Here's how the part is built. I have some questions about the finished solid (model axes, mm). A direction names the side the tool comes from. Round coordinates to 2 decimals unless told otherwise and drop trailing zeros. Loops run counter-clockwise (first coordinate to the right, second up) from the corner with the lowest first, then second, coordinate; pieces in that order, holes last. Notation, with made-up numbers: (2.25, 19.5) -> (24.25, 19.5) arc R33 ccw to (24.25, 54.5) -> close; hole circle Ø3 at (88, -16.75). An arc over 180 degrees is marked (long way). Use one line per item in the form item = value. Start each with the question number.
Item 1: If we section it at A-A (y = 0): Write out the boundary of the cut face in (x, z) (3 decimals), then the cut area to 3 significant figures.
Item 2: If we section it at D-D (y = 18): Write out the boundary of the cut face in (x, z), then the cut area to 3 significant figures.
Item 3: I'm going to push flat-ended pins straight in: pin 1 Ø14 at (x, y) = (2, 1) entering from +Z; pin 2 Ø5 at (x, z) = (-7, 14) entering from -Y; pin 3 Ø12 at (x, y) = (-10.5, 3.5) entering from +Z; pin 4 Ø10 at (y, z) = (7.5, 9) entering from +X. Where does each tip first touch, or does it pass through?
Item 4: If we section it at B-B (z = 10.5): Write out the boundary of the cut face in (x, y).
Item 5: Thinking about a two-plate mould opening in Z: for faces 1 (the face through (0, -6, 0)), 2 (the face through (0, 25, 14)), 3 (the face through (18.567, 21.204, 19.586)), which applies, released by +Z, released by -Z, zero draft, split by the parting line, or undercut?
Item 6: If we section it at C-C (x = -20): Write out the boundary of the cut face in (y, z), then the cut area to 3 significant figures.
Item 7: For faces 4 (the face through (-24.57, -24.55, 2.79)), 5 (the face through (0, 17.3, 17)), which set-ups out of +Z, -Z, +X, -X, +Y, -Y let a thin tool reach every point of the face, with its end or its side?
Item 8: If I drill on L1, parallel to X at y = 20.5, z = 10.5; L2, parallel to X at y = 0, z = 4.3; L3, parallel to X at y = 9, z = 0.8 (3 decimals), over which ranges is the centre line in solid material (lowest first)? Write a range as [from, to].
Autodesk Fusion 360 part; units mm, degrees
sketch "Sketch1" plane through (0, 0, 0) normal (0, 0, 1) x (1, 0, 0)
  line L0 (25, 25) -> (-25, 25)
  line L1 (-25, 25) -> (-25, -25)
  line L2 (-25, -25) -> (25, -25)
  line L3 (25, -25) -> (25, 25)
  line L4 (25, 25) -> (-25, -25) construction
  line L5 (-25, 25) -> (25, -25) construction
  dimension "d1" = 50
  dimension "d2" = 50
extrude "Extrude1" add sketch "Sketch1" along normal blind 5.5
sketch "Sketch2" plane through (0, 0, 5.5) normal (0, 0, 1) x (-1, 0, 0)
  line L0 (-25, 25) -> (-25, -25)
  line L1 (-25, -25) -> (25, -25)
  line L2 (25, -25) -> (25, 25)
  line L3 (25, 25) -> (-25, 25)
  line L4 (25, -25) -> (-25, -25)
  line L5 (-25, -25) -> (-25, -17.3)
  line L6 (-25, -17.3) -> (25, -17.3)
  line L7 (25, -17.3) -> (25, -25)
  dimension "d11" = 7.7
  dimension "d12" = 50
extrude "Extrude2" add sketch "Sketch2" along normal blind 20 contours L0 L1 L2 L4 L5 L6 L7
sketch "Sketch3" plane through (0, 0, 5.5) normal (0, 0, 1) x (-1, 0, 0)
  line L0 (-25, -17.3) -> (25, -17.3)
  line L1 (25, -17.3) -> (25, 25)
  line L2 (25, 25) -> (-25, 25)
  line L3 (-25, 25) -> (-25, -17.3)
  circle A0 centre (0, 0) radius 14
  dimension "d15" = 28
sketch "Sketch4" plane through (0, 0, 5.5) normal (0, 0, 1) x (-1, 0, 0)
fillet "Fillet1" radius 2.5 1 edges at (0, 17.3, 5.5)
fillet "Fillet2" radius 3 1 edges at (0, 25, 0)
fillet "Fillet3" radius 1.5 4 edges at (25, -25, 2.75) (-25, -25, 2.75) (25, 21.15, 25.5) (-25, 21.15, 25.5)
extrude "Extrude3" cut sketch "Sketch3" against normal blind 2 contours A0
sketch "Sketch5" plane through (0, 0, 5.5) normal (0, 0, 1) x (-1, 0, 0)
  circle A0 centre (0, 0) radius 14
  arc A1 (25, 23.5) -> (23.5, 25) centre (23.5, 23.5) ccw
  line L0 (23.5, 25) -> (-23.5, 25)
  arc A2 (-23.5, 25) -> (-25, 23.5) centre (-23.5, 23.5) ccw
  line L1 (-25, 23.5) -> (-25, -14.8)
  line L2 (-25, -14.8) -> (25, -14.8)
  line L3 (25, -14.8) -> (25, 23.5)
  circle A3 centre (0, 0) radius 9 construction
  point P0 (0, -9)
  dimension "d24" = 18
hole "Hole1" at (0, 0, 5.5) direction (0, 0, -1) diameter 6.1 depth 10 tip angle 118
hole "Hole2" at (0, 9, 5.5) direction (0, 0, -1) diameter 2.93 depth 10 tip angle 118
pattern_circular "C-Pattern1" count 4 over 360 about axis through (0, 0, 1.75) along (0, 0, 1) of "Hole2"
hole "Hole3" at (-20, 17.3, 20.5) direction (0, 1, 0) diameter 3.4 depth 10 tip angle 118
hole "Hole4" at (-20, 17.3, 10.5) direction (0, 1, 0) diameter 3.4 depth 10 tip angle 118
hole "Hole5" at (20, 17.3, 20.5) direction (0, 1, 0) diameter 3.4 depth 10 tip angle 118
hole "Hole6" at (20, 17.3, 10.5) direction (0, 1, 0) diameter 3.4 depth 10 tip angle 118
equation "Base_Feature_1 = 50 mm"
equation "Width_Feature_1 = 50 mm"
equation "thickness_Feature_1 = 5.5 mm"
equation "Base_Feature_2 = 50 mm"
equation "Height_Feature_2 = 20 mm"
equation "Thickness_Feature_2 = 7.7 mm"
equation "d11 = Thickness_Feature_2"
equation "d12 = Base_Feature_2"
equation "d13 = Height_Feature_2"
equation "Feature_2_Edge = 5 mm"
equation "Feature_2_Top = 5.0 mm"
equation "Feat_2_Left_Holes_Xpos = Feature_2_Edge"
equation "Feat_2_Right_Holes_xpos = Base_Feature_2 - Feature_2_Edge"
equation "motor_hole = 6.1 mm"
equation "Feature_1_Motor_Hole = 6.1 mm"
equation "Feature_1_Motor_Mount_Hole_Size = 3 mm"
Values found:
q1.outline = (-25, 0) -> (-10.465, 0) -> (-10.465, 3.5) -> (-14, 3.5) -> (-14, 5.5) -> (-25, 5.5) -> close; (-7.535, 0) -> (-3.05, 0) -> (-3.05, 3.5) -> (-7.535, 3.5) -> close; (3.05, 0) -> (7.535, 0) -> (7.535, 3.5) -> (3.05, 3.5) -> close; (10.465, 0) -> (25, 0) -> (25, 5.5) -> (14, 5.5) -> (14, 3.5) -> (10.465, 3.5) -> close
q1.area = 177 mm2
q2.outline = (-25, 0) -> (25, 0) -> (25, 24) arc R1.5 ccw to (23.5, 25.5) -> (-23.5, 25.5) arc R1.5 ccw to (-25, 24) -> close; hole circle Ø3.4 at (-20, 10.5); hole circle Ø3.4 at (-20, 20.5); hole circle Ø3.4 at (20, 10.5); hole circle Ø3.4 at (20, 20.5)
q2.area = 1,240 mm2
q3.pin_1 = 3.5
q3.pin_2 = 17.3
q3.pin_3 = 5.5
q3.pin_4 = 25
q4.outline = (-25, 17.3) -> (-21.7, 17.3) -> (-21.7, 25) -> (-25, 25) -> close; (-18.3, 17.3) -> (18.3, 17.3) -> (18.3, 25) -> (-18.3, 25) -> close; (21.7, 17.3) -> (25, 17.3) -> (25, 25) -> (21.7, 25) -> close
q5.face_1 = released by -Z
q5.face_2 = zero draft
q5.face_3 = undercut
q6.outline = (-25, 0) -> (22, 0) arc R3 ccw to (25, 3) -> (25, 8.8) -> (17.3, 8.8) -> (17.3, 8) arc R2.5 cw to (14.8, 5.5) -> (-25, 5.5) -> close; (17.3, 12.2) -> (25, 12.2) -> (25, 18.8) -> (17.3, 18.8) -> close; (17.3, 22.2) -> (25, 22.2) -> (25, 25.5) -> (17.3, 25.5) -> close
q6.area = 376 mm2
q7.face_4 = +Z, -Z, -X, -Y
q7.face_5 = +Z, +X, -X, -Y
q8.L1 = [-25, -21.7], [-18.3, 18.3], [21.7, 25]
q8.L2 = [-25, -14], [14, 25]
q8.L3 = [-25, -1.465], [1.465, 25]
